Geometry check sheet. Reference: the model listing, model coordinates, mm. Face numbers are marked on the shaded views. Round coordinates to 2 decimals unless told otherwise and drop trailing zeros. Write each loop counter-clockwise with the first axis right and the second up, starting at its lowest first coordinate (ties: lowest second). Pieces come first, ordered by that corner, then holes. Notation, with made-up numbers: M 43,11 L 73,11 A21 ccw 73,24 Z; hole C 84.25,35 d5. An arc over 180 degrees is marked long. Put each result on its own line as item: value. Start each with the question number.
(1) Mould release check, pull along Y, two halves, no side actions. Record for the marked faces 1, 2 and 3: pulls with the +Y half, pulls with the -Y half, needs draft (parallel to the pull), parting line crosses it, or undercut.
(2) Gauge pin test, flat ends, axial feed: pin 1 (1.5 mm diameter, centred on x = -9.5, y = -29, fed in from -Z); pin 2 (3 mm diameter, centred on y = -1.5, z = 1.5, fed in from +X); pin 3 (3 mm diameter, centred on y = -32.5, z = 2, fed in from +X) (3 decimals); pin 4 (2 mm diameter, centred on y = -12.5, z = 1, fed in from -X). Record the tip position at first contact, or that the pin passes through.
(3) Material ranges on probe 1 along X at (y, z) = (12, 5); probe 2 along X at (y, z) = (4, 2.5); probe 3 along Y at (x, z) = (-8, 1.75), recorded low to high.
(4) Section check B-B on x = 0. Count the separate pieces of the cut face and the enclosed holes in it, then the cut area to 3 significant figures.
(5) Section check A-A on y = 0. Record the cut outline in (x, z).
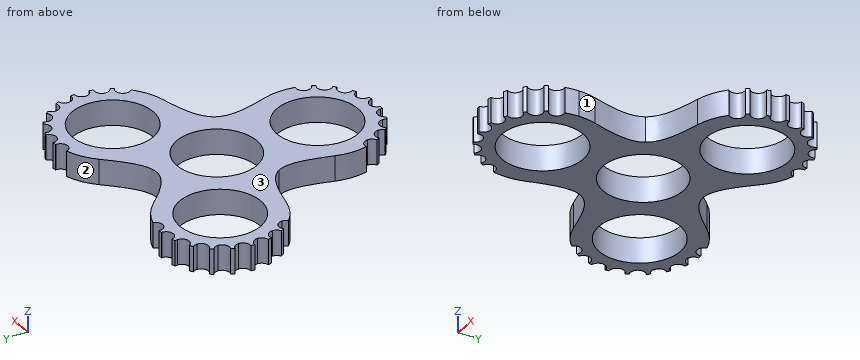
from build123d import *

# Parameters (mm, degrees)
F0_R     = 11.25
F0_R_2   = 11.1
F1_DEPTH = 7


with BuildPart() as f1:
    # F0 (on Top) → F1 (new body)
    with BuildSketch(Plane.XY):
        with BuildLine():
            ThreePointArc((-7.748711, 14), (-8.896077, 20.045379), (-12.178604, 25.25))
            ThreePointArc((-12.178604, 25.25), (-15.509523, 27.995592), (-19.43857, 29.783299))
            ThreePointArc((-19.43857, 29.783299), (-21.730813, 28.279712), (-23.37056, 30.476615))
            ThreePointArc((-23.37056, 30.476615), (-23.888766, 30.496073), (-24.407327, 30.499238))
            ThreePointArc((-24.407327, 30.499238), (-24.403627, 30.429082), (-24.402393, 30.35884))
            ThreePointArc((-24.402393, 30.35884), (-26.211143, 28.368005), (-28.365817, 29.978093))
            ThreePointArc((-28.365817, 29.978093), (-28.86589, 29.840823), (-29.361403, 29.687906))
            ThreePointArc((-29.361403, 29.687906), (-29.257095, 29.327562), (-29.221913, 28.954078))
            ThreePointArc((-29.221913, 28.954078), (-30.730036, 27.015508), (-32.97997, 28.00054))
            ThreePointArc((-32.97997, 28.00054), (-33.41562, 27.719249), (-33.842216, 27.424406))
            ThreePointArc((-33.842216, 27.424406), (-33.510815, 26.833108), (-33.39595, 26.165076))
            ThreePointArc((-33.39595, 26.165076), (-34.614896, 24.323893), (-36.785904, 24.727012))
            ThreePointArc((-36.785904, 24.727012), (-37.116805, 24.327737), (-37.434996, 23.918261))
            ThreePointArc((-37.434996, 23.918261), (-36.776559, 23.19703), (-36.53813, 22.25))
            ThreePointArc((-36.53813, 22.25), (-37.48608, 20.549062), (-39.431319, 20.460527))
            ThreePointArc((-39.431319, 20.460527), (-39.626841, 19.980228), (-39.807173, 19.494021))
            ThreePointArc((-39.807173, 19.494021), (-38.760591, 18.775238), (-38.357595, 17.571254))
            ThreePointArc((-38.357595, 17.571254), (-39.059036, 16.050154), (-40.67134, 15.596016))
            ThreePointArc((-40.67134, 15.596016), (-40.713384, 15.079152), (-40.739164, 14.561221))
            ThreePointArc((-40.739164, 14.561221), (-39.29066, 13.994843), (-38.685924, 12.56193))
            ThreePointArc((-38.685924, 12.56193), (-39.171083, 11.256075), (-40.391182, 10.583768))
            ThreePointArc((-40.391182, 10.583768), (-40.275855, 10.078183), (-40.144698, 9.576472))
            ThreePointArc((-40.144698, 9.576472), (-38.331679, 9.314212), (-37.492724, 7.685723))
            ThreePointArc((-37.492724, 7.685723), (-37.796862, 6.625509), (-38.616778, 5.887747))
            ThreePointArc((-38.616778, 5.887747), (-38.354757, 5.440241), (-38.078803, 5.001191))
            ThreePointArc((-38.078803, 5.001191), (-35.988644, 5.180162), (-34.888445, 3.394004))
            ThreePointArc((-34.888445, 3.394004), (-35.051037, 2.604109), (-35.512379, 1.942646))
            ThreePointArc((-35.512379, 1.942646), (-31.999656, -0.566155), (-27.956443, -2.07802))
            ThreePointArc((-27.956443, -2.07802), (-13.975629, 1.088231), (-7.748711, 14))
        make_face()
        with Locations((-24.248711, 14)):
            Circle(F0_R, mode=Mode.SUBTRACT)
        with BuildLine():
            ThreePointArc((27.956443, -2.07802), (9.959292, 5.75), (12.178604, 25.25))
            add(Edge.make_bspline(
                [(0, 16.75), (4.085687, 16.75), (8.171373, 20.950648), (12.178604, 25.25)],
                knots=[14.851545, 14.851545, 14.851545, 14.851545, 29.70309, 29.70309, 29.70309, 29.70309], degree=3))
            add(Edge.make_bspline(
                [(-12.178604, 25.25), (-8.171373, 20.950648), (-4.085687, 16.75), (0, 16.75)],
                knots=[0, 0, 0, 0, 14.851545, 14.851545, 14.851545, 14.851545], degree=3))
            ThreePointArc((-12.178604, 25.25), (-8.896077, 20.045379), (-7.748711, 14))
            ThreePointArc((-7.748711, 14), (-13.975629, 1.088231), (-27.956443, -2.07802))
            add(Edge.make_bspline(
                [(-27.956443, -2.07802), (-22.22948, -3.398708), (-16.548769, -4.836692), (-14.505926, -8.375)],
                knots=[0, 0, 0, 0, 14.851545, 14.851545, 14.851545, 14.851545], degree=3))
            add(Edge.make_bspline(
                [(-14.505926, -8.375), (-12.463082, -11.913308), (-14.058107, -17.551941), (-15.77784, -23.17198)],
                knots=[14.851545, 14.851545, 14.851545, 14.851545, 29.70309, 29.70309, 29.70309, 29.70309], degree=3))
            ThreePointArc((-15.77784, -23.17198), (0, -11.5), (15.77784, -23.17198))
            add(Edge.make_bspline(
                [(14.505926, -8.375), (12.463082, -11.913308), (14.058107, -17.551941), (15.77784, -23.17198)],
                knots=[14.851545, 14.851545, 14.851545, 14.851545, 29.70309, 29.70309, 29.70309, 29.70309], degree=3))
            add(Edge.make_bspline(
                [(27.956443, -2.07802), (22.22948, -3.398708), (16.548769, -4.836692), (14.505926, -8.375)],
                knots=[0, 0, 0, 0, 14.851545, 14.851545, 14.851545, 14.851545], degree=3))
        make_face()
        Circle(F0_R_2, mode=Mode.SUBTRACT)
        with BuildLine():
            ThreePointArc((19.43857, 29.783299), (15.509523, 27.995592), (12.178604, 25.25))
            ThreePointArc((12.178604, 25.25), (9.959292, 5.75), (27.956443, -2.07802))
            ThreePointArc((27.956443, -2.07802), (31.999656, -0.566155), (35.512379, 1.942646))
            ThreePointArc((35.512379, 1.942646), (35.356356, 4.67958), (38.078803, 5.001191))
            ThreePointArc((38.078803, 5.001191), (38.354757, 5.440241), (38.616778, 5.887747))
            ThreePointArc((38.616778, 5.887747), (37.644965, 8.45109), (40.144698, 9.576472))
            ThreePointArc((40.144698, 9.576472), (40.275855, 10.078183), (40.391182, 10.583768))
            ThreePointArc((40.391182, 10.583768), (38.693534, 12.736242), (40.739164, 14.561221))
            ThreePointArc((40.739164, 14.561221), (40.713384, 15.079152), (40.67134, 15.596016))
            ThreePointArc((40.67134, 15.596016), (38.405003, 17.138374), (39.807173, 19.494021))
            ThreePointArc((39.807173, 19.494021), (39.626841, 19.980228), (39.431319, 20.460527))
            ThreePointArc((39.431319, 20.460527), (36.80608, 21.25), (37.434996, 23.918261))
            ThreePointArc((37.434996, 23.918261), (37.116805, 24.327737), (36.785904, 24.727012))
            ThreePointArc((36.785904, 24.727012), (34.044769, 24.690521), (33.842216, 27.424406))
            ThreePointArc((33.842216, 27.424406), (33.41562, 27.719249), (32.97997, 28.00054))
            ThreePointArc((32.97997, 28.00054), (30.376676, 27.141463), (29.361403, 29.687906))
            ThreePointArc((29.361403, 29.687906), (28.86589, 29.840823), (28.365817, 29.978093))
            ThreePointArc((28.365817, 29.978093), (26.141341, 28.37595), (24.407327, 30.499238))
            ThreePointArc((24.407327, 30.499238), (23.888766, 30.496073), (23.37056, 30.476615))
            ThreePointArc((23.37056, 30.476615), (23.380275, 30.363156), (23.383516, 30.249328))
            ThreePointArc((23.383516, 30.249328), (21.618151, 28.263139), (19.43857, 29.783299))
        make_face()
        with Locations((24.248711, 14)):
            Circle(F0_R, mode=Mode.SUBTRACT)
        with BuildLine():
            ThreePointArc((16.5, -28), (16.318461, -25.559135), (15.77784, -23.17198))
            ThreePointArc((15.77784, -23.17198), (0, -11.5), (-15.77784, -23.17198))
            ThreePointArc((-15.77784, -23.17198), (-16.490132, -27.429437), (-16.073809, -31.725945))
            ThreePointArc((-16.073809, -31.725945), (-14.308634, -32.04056), (-13.504928, -33.643332))
            ThreePointArc((-13.504928, -33.643332), (-13.832599, -34.74029), (-14.708243, -35.477806))
            ThreePointArc((-14.708243, -35.477806), (-14.465991, -35.936315), (-14.209451, -36.386984))
            ThreePointArc((-14.209451, -36.386984), (-12.151778, -36.27846), (-11.09033, -38.044564))
            ThreePointArc((-11.09033, -38.044564), (-11.270591, -38.874353), (-11.778881, -39.554564))
            ThreePointArc((-11.778881, -39.554564), (-11.409965, -39.919005), (-11.029779, -40.271673))
            ThreePointArc((-11.029779, -40.271673), (-8.805048, -39.627685), (-7.464011, -41.516009))
            ThreePointArc((-7.464011, -41.516009), (-7.539221, -42.059316), (-7.759194, -42.561762))
            ThreePointArc((-7.759194, -42.561762), (-7.297763, -42.7984), (-6.829124, -43.020422))
            ThreePointArc((-6.829124, -43.020422), (-4.597611, -41.769739), (-2.961646, -43.73633))
            ThreePointArc((-2.961646, -43.73633), (-2.976607, -43.980508), (-3.021269, -44.221034))
            ThreePointArc((-3.021269, -44.221034), (-2.510036, -44.307965), (-1.996324, -44.378788))
            ThreePointArc((-1.996324, -44.378788), (0, -42.5), (1.996324, -44.378788))
            ThreePointArc((1.996324, -44.378788), (2.510036, -44.307965), (3.021269, -44.221034))
            ThreePointArc((3.021269, -44.221034), (4.360234, -41.828896), (6.829124, -43.020422))
            ThreePointArc((6.829124, -43.020422), (7.297763, -42.7984), (7.759194, -42.561762))
            ThreePointArc((7.759194, -42.561762), (8.316858, -39.877705), (11.029779, -40.271673))
            ThreePointArc((11.029779, -40.271673), (11.409965, -39.919005), (11.778881, -39.554564))
            ThreePointArc((11.778881, -39.554564), (11.503623, -36.827041), (14.209451, -36.386984))
            ThreePointArc((14.209451, -36.386984), (14.465991, -35.936315), (14.708243, -35.477806))
            ThreePointArc((14.708243, -35.477806), (13.625543, -32.959292), (16.073809, -31.725945))
            ThreePointArc((16.073809, -31.725945), (16.393106, -29.87512), (16.5, -28))
        make_face()
        with Locations((0, -28)):
            Circle(F0_R, mode=Mode.SUBTRACT)
    extrude(amount=F1_DEPTH)


solid = f1.part
Answers follow:
1. face 1: undercut
1. face 2: pulls with the +Y half
1. face 3: needs draft
2. pin 1: passes through
2. pin 2: stops at x = 32.98
2. pin 3: stops at x = 16.225
2. pin 4: stops at x = -13.59
3. probe 1: x = -38.77 to -35.32, -13.18 to 13.18, 35.32 to 38.77
3. probe 2: x = -34.98 to -29.4, -19.09 to -10.35, 10.35 to 19.09, 29.4 to 34.98
3. probe 3: y = -40.15 to -35.91, -20.09 to -7.69, 7.69 to 21
4. separate pieces: 3
4. enclosed holes: 0
4. area: 102 mm^2
5. outline: M -32.98,0 L -11.1,0 L -11.1,7 L -32.98,7 Z; M 11.1,0 L 32.98,0 L 32.98,7 L 11.1,7 Z
